```python
from build123d import *

# Parameters (mm, degrees)
F0_W     = 135
F0_H     = 30
F1_DEPTH = 15
F2_W     = 113
F2_H     = 5
F3_DEPTH = 4
F4_W     = 5
F4_H     = 4
F5_DEPTH = 4


with BuildPart() as f1:
    # F0 (on Front) → F1 (new body)
    with BuildSketch(Plane.XZ):
        with Locations((0, 15)):
            Rectangle(F0_W, F0_H)
    extrude(amount=F1_DEPTH)

    # F2 (on face) → F3 (cut)
    with BuildSketch(Plane.XY.offset(30)):
        with Locations((0, -5.95)):
            Rectangle(F2_W, F2_H)
    extrude(amount=-F3_DEPTH, mode=Mode.SUBTRACT)

    # F4 (on face) → F5 (cut)
    with BuildSketch(Plane.XY.offset(30)):
        with Locations((61.5, -13)):
            Rectangle(F4_W, F4_H)
        with Locations((-61.5, -13)):
            Rectangle(F4_W, F4_H)
    extrude(amount=-F5_DEPTH, mode=Mode.SUBTRACT)


solid = f1.part
```
CAD build for the part. Positions are in the model's coordinates, mm. A direction names the side the tool comes from. Coordinates: 2 decimals unless noted, no trailing zeros. Loops run counter-clockwise (first coordinate to the right, second up) from the corner with the lowest first, then second, coordinate; pieces in that order, holes last. Notation, with made-up numbers: (68.5, -23.75) - (103.5, -23.75) arc R27 cw to (103.5, 8.25) - close; hole circle Ø1 at (4, -40). An arc over 180 degrees is marked (long way). Return JSON: item names as keys, results as strings.
1. Mould opens along X. For faces 1 (the flat face through (-67.5, -7, 15)), 2 (the flat face through (-1, 0, 15)), 3 (the flat face through (67.5, -7, 15)), 4 (the flat face through (61, -13, 26)) say: released by +X, released by -X, zero draft, split by the parting line, or undercut.
Result:
{"face 1": "released by -X", "face 2": "zero draft", "face 3": "released by +X", "face 4": "undercut"}
2. 3-axis set-ups, long thin cutter, end or side, ignore diameter. For faces 5 (the flat face through (-1, -3.45, 28)), 6 (the flat face through (-1, -7, 0)), 7 (the flat face through (-62, -13, 26)): which of +Z, -Z, +X, -X, +Y, -Y reach the whole face in a straight line?
Result:
{"face 5": "+Z", "face 6": "-Z, +X, -X, +Y, -Y", "face 7": "+Z, -Y"}
3. Probe L1, parallel to Y at x = -33, z = 28.75; L2, parallel to Z at x = 43, y = -5.25; L3, parallel to Y at x = -61, z = 26.5. List the from-to ranges inside material, lowest first. Write a range as from..to.
Result:
{"L1": "y = -15..-8.45, -3.45..0", "L2": "z = 0..26", "L3": "y = -11..0"}
4. Band-saw the part on B-B (y = -6). Give the cut face in (x, z).
Result:
{"outline": "(-67.5, 0) - (67.5, 0) - (67.5, 30) - (56.5, 30) - (56.5, 26) - (-56.5, 26) - (-56.5, 30) - (-67.5, 30) - close"}
5. Band-saw the part on A-A (x = -14). Give the cut face in (y, z), and give its area (3 significant figures).
Result:
{"outline": "(-15, 0) - (0, 0) - (0, 30) - (-3.45, 30) - (-3.45, 26) - (-8.45, 26) - (-8.45, 30) - (-15, 30) - close", "area": "430 mm2"}
6. Drop flat-ended pins along their axis: pin 1 (3 mm diameter, centred on x = -61.5, y = -13.5, fed in from +Z); pin 2 (1.2 mm diameter, centred on x = -61.5, z = 27.5, fed in from -Y). Give the stop position or say it passes through.
Result:
{"pin 1": "stops at z = 26", "pin 2": "stops at y = -11"}
